Build history of the part. All positions in model axes, mm. Face numbers are marked on the shaded views. Round coordinates to 2 decimals unless told otherwise and drop trailing zeros. Loops run counter-clockwise (first coordinate to the right, second up) from the corner with the lowest first, then second, coordinate; pieces in that order, holes last. Notation, with made-up numbers: (34.5, 32) - (79.5, 32) arc R23 ccw to (79.5, 43) - close; hole circle Ø7 at (77, 76.5). An arc over 180 degrees is marked (long way). Use one line per item in the form item = value. Start each with the question number.
Q1. Pin check, flat tips, straight feed: pin 1 (10 mm diameter, centred on x = -4, z = -7.5, fed in from -Y); pin 2 (1.5 mm diameter, centred on y = 2, z = -9, fed in from -X). Stop position of each tip, or through.
Q2. Mould opens along X. For the marked faces 1 and 2 say: released by +X, released by -X, zero draft, split by the parting line, or undercut.
Q3. Saw through at B-B (z = 0). Give the cut face in (x, y), then the cut area to 3 significant figures.
Q4. Drill centre lines: line 1 (X direction, y = 1.7, z = 0); line 2 (Y direction, x = 7.5, z = 7); line 3 (X direction, y = 2, z = -6). Where is each one in solid material? Low to high.
Q5. Saw through at C-C (y = 1.25). Give the cut face in (x, z).
Q6. Saw through at A-A (x = 0). Give the cut face in (y, z), then the cut area to 3 significant figures.
```python
from build123d import *


with BuildPart() as part:
    # Esquisse2 → Révolution1 (revolve)
    with BuildSketch(Plane.XY, mode=Mode.PRIVATE) as r_volution1_sk:
        with BuildLine():
            Line((0, 5.5), (21, 5.5))
            ThreePointArc((21, 5.5), (22.414213562, 4.914213562), (23, 3.5))
            Line((23, 3.5), (23, 2.5))
            Line((23, 2.5), (19, 2.5))
            Line((19, 2.5), (19, 0))
            Line((19, 0), (17, 0))
            Line((17, 0), (17, 2.5))
            Line((17, 2.5), (0, 2.5))
            Line((0, 2.5), (0, 5.5))
        make_face()
    revolve(r_volution1_sk.sketch.rotate(Axis((0, 31.915652174, 0), (0, -1, 0)), 90), axis=Axis((0, 31.915652174, 0), (0, -1, 0)))


solid = part.part
```
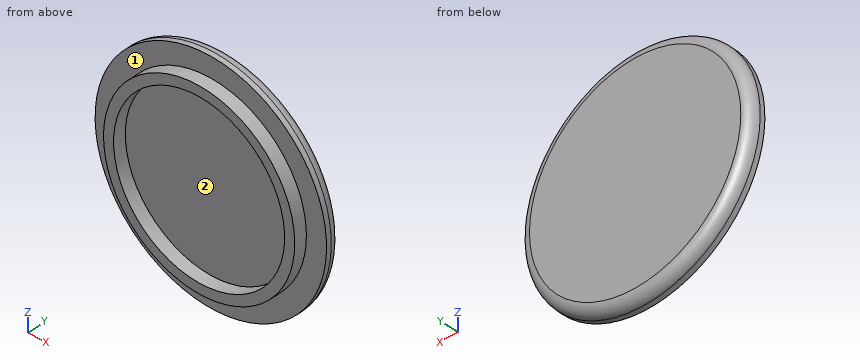
Report:
q1.pin_1 = 2.5
q1.pin_2 = -21.4
q2.face_1 = zero draft
q2.face_2 = undercut
q3.outline = (-23, 2.5) - (-19, 2.5) - (-19, 0) - (-17, 0) - (-17, 2.5) - (17, 2.5) - (17, 0) - (19, 0) - (19, 2.5) - (23, 2.5) - (23, 3.5) arc R2 ccw to (21, 5.5) - (-21, 5.5) arc R2 ccw to (-23, 3.5) - close
q3.area = 146 mm²
q4.line_1 = -19 to -17, 17 to 19
q4.line_2 = 2.5 to 5.5
q4.line_3 = -18.03 to -15.91, 15.91 to 18.03
q5.outline = circle Ø38 at (0, 0); hole circle Ø34 at (0, 0)
q6.outline = (0, -19) - (2.5, -19) - (2.5, -23) - (3.5, -23) arc R2 ccw to (5.5, -21) - (5.5, 21) arc R2 ccw to (3.5, 23) - (2.5, 23) - (2.5, 19) - (0, 19) - (0, 17) - (2.5, 17) - (2.5, -17) - (0, -17) - close
q6.area = 146 mm²
